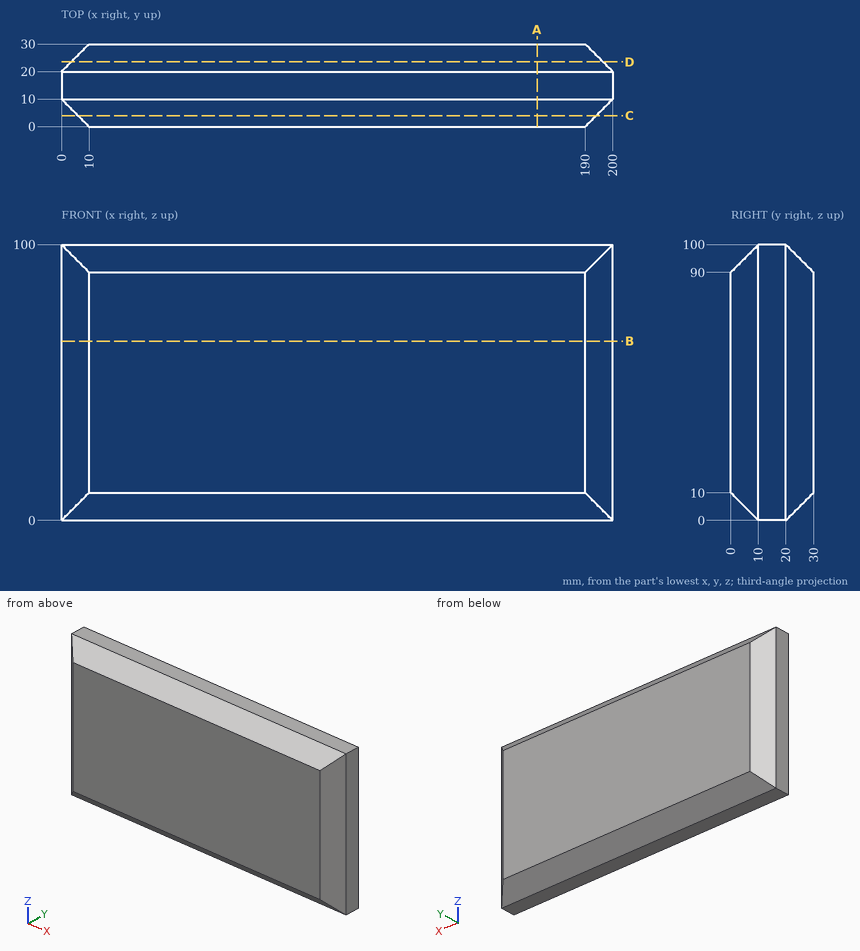
Geometry: see drawing. Coordinates: mm, zero at the bounding-box minimum. Coordinates: 2 decimals unless noted, no trailing zeros. Loops run counter-clockwise (first coordinate to the right, second up) from the corner with the lowest first, then second, coordinate; pieces in that order, holes last.
(1) Section A-A on x = 172.5. Return the cut outline in (y, z), then the cut area to 3 significant figures.
(2) Section C-C on y = 4. Return the cut outline in (x, z), then the cut area to 3 significant figures.
(3) Section B-B on z = 65. Return the cut outline in (x, y).
(4) Section D-D on y = 23.5. Return the cut outline in (x, z).
(5) Material intervals for probe 1 along Z at (x, y) = (21, 9.5); probe 2 along Z at (x, y) = (154.5, 3); probe 3 along X at (y, z) = (26.5, 61), sorted ascending.
(6) First-contact query: pin 1 Ø4 at (y, z) = (24.5, 69) entering from -X; pin 2 Ø1 at (y, z) = (21, 22.5) entering from +X; pin 3 Ø4 at (y, z) = (23.5, 44) entering from -X. Flat tips, straight axial feed; report the tip coordinate or a pass-through.
Data:
1. outline: (0, 10) - (10, 0) - (20, 0) - (30, 10) - (30, 90) - (20, 100) - (10, 100) - (0, 90) - close
1. area: 2,800 mm2
2. outline: (6, 6) - (194, 6) - (194, 94) - (6, 94) - close
2. area: 16,500 mm2
3. outline: (0, 10) - (10, 0) - (190, 0) - (200, 10) - (200, 20) - (190, 30) - (10, 30) - (0, 20) - close
4. outline: (3.5, 3.5) - (196.5, 3.5) - (196.5, 96.5) - (3.5, 96.5) - close
5. probe 1: z = 0.5 to 99.5
5. probe 2: z = 7 to 93
5. probe 3: x = 6.5 to 193.5
6. pin 1: stops at x = 2.5
6. pin 2: stops at x = 199.5
6. pin 3: stops at x = 1.5
